Geometry check sheet. Reference: the model listing, model coordinates, mm. Face numbers are marked on the shaded views. A direction names the side the tool comes from. Give positions to 0.01 mm unless a question says otherwise; leave off trailing zeros. Loops run counter-clockwise (first coordinate to the right, second up) from the corner with the lowest first, then second, coordinate; pieces in that order, holes last. Notation, with made-up numbers: (2, 66) -> (21, 66) arc R17 cw to (21, 99) -> close; hole circle Ø4 at (89.5, -14.75). An arc over 180 degrees is marked (long way). Answer as a JSON object with one key per item and string values.
from build123d import *

# Parameters (mm, degrees)
SKETCH2_W           = 9.2
SKETCH2_H           = 22.44
SKETCH2_R           = 1.6
BOSS_EXTRUDE2_DEPTH = 3
SKETCH4_W           = 2
SKETCH4_H           = 22.44
BOSS_EXTRUDE3_DEPTH = 18
FILLET1_R           = 2
SKETCH5_R           = 1.6
CUT_EXTRUDE1_DEPTH  = 18


with BuildPart() as part:
    # Sketch2 → Boss-Extrude2 (new body)
    with BuildSketch(Plane(origin=(0, 0, 0), x_dir=(1, 0, 0), z_dir=(0, 1, 0))):
        with Locations((4.6, 11.22)):
            Rectangle(SKETCH2_W, SKETCH2_H)
        with Locations((5.6, 16.22)):
            Circle(SKETCH2_R, mode=Mode.SUBTRACT)
        with Locations((5.6, 6.22)):
            Circle(SKETCH2_R, mode=Mode.SUBTRACT)
    extrude(amount=BOSS_EXTRUDE2_DEPTH)

    # Sketch4 → Boss-Extrude3 (add)
    with BuildSketch(Plane(origin=(0, 3, 0), x_dir=(1, 0, 0), z_dir=(0, 1, 0))):
        with Locations((1, 11.22)):
            Rectangle(SKETCH4_W, SKETCH4_H)
    extrude(amount=BOSS_EXTRUDE3_DEPTH)

    # Fillet1
    fillet1_edges = [part.edges().sort_by_distance(p)[0] for p in [
        (0, 0, -11.22),
    ]]
    fillet(fillet1_edges, radius=FILLET1_R)

    # Sketch5 → Cut-Extrude1 (cut)
    with BuildSketch(Plane(origin=(2, 0, 0), x_dir=(0, 0, -1), z_dir=(1, 0, 0))):
        with Locations((2.42, 16)):
            Circle(SKETCH5_R)
        with Locations((20.02, 16)):
            Circle(SKETCH5_R)
    extrude(amount=-CUT_EXTRUDE1_DEPTH, mode=Mode.SUBTRACT)


solid = part.part
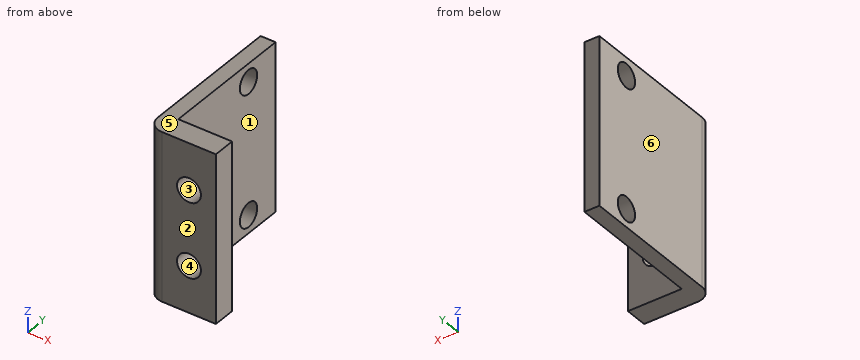
1) Section check D-D on z = -16.22. Record the cut outline in (x, y), plus the area to 3 significant figures.
Geometry check:
{"outline": "(0, 2) arc R2 ccw to (2, 0) -> (4, 0) -> (4, 3) -> (2, 3) -> (2, 21) -> (0, 21) -> close; (7.2, 0) -> (9.2, 0) -> (9.2, 3) -> (7.2, 3) -> close", "area": "53.1 mm2"}
2) Depth check by flat-ended pin: P1, Ø3, axis at x = 6, z = -9, coming from the +Y side; P2, Ø3, axis at y = 10.5, z = -13.5, coming from the +X side. Enter the tip coordinate at first touch or a pass-through.
Geometry check:
{"P1": "stops at y = 3", "P2": "stops at x = 2"}
3) Section check C-C on y = 16. Record the cut outline in (x, z), plus the area to 3 significant figures.
Geometry check:
{"outline": "(0, -22.44) -> (2, -22.44) -> (2, -21.62) -> (0, -21.62) -> close; (0, -18.42) -> (2, -18.42) -> (2, -4.02) -> (0, -4.02) -> close; (0, -0.82) -> (2, -0.82) -> (2, 0) -> (0, 0) -> close", "area": "32.1 mm2"}
4) Section check B-B on x = 5.6. Record the cut outline in (y, z), plus the area to 3 significant figures.
Geometry check:
{"outline": "(0, -22.44) -> (3, -22.44) -> (3, -17.82) -> (0, -17.82) -> close; (0, -14.62) -> (3, -14.62) -> (3, -7.82) -> (0, -7.82) -> close; (0, -4.62) -> (3, -4.62) -> (3, 0) -> (0, 0) -> close", "area": "48.1 mm2"}
5) Draft check along X on the marked faces 3, 4, 5 and 6. Enter one of: pulls with the +X half, pulls with the -X half, needs draft (parallel to the pull), parting line crosses it, or undercut.
Geometry check:
{"face 3": "undercut", "face 4": "undercut", "face 5": "needs draft", "face 6": "pulls with the -X half"}
6) Material ranges on line 1 along Z through (x, y) = (5.6, 1.8); line 2 along X through (y, z) = (2.35, -16.22); line 3 along X through (y, z) = (14, -11.25), recorded low to high. Write a range as from..to.
Geometry check:
{"line 1": "z = -22.44..-17.82, -14.62..-7.82, -4.62..0", "line 2": "x = 0..4, 7.2..9.2", "line 3": "x = 0..2"}
7) Tool access check on the marked faces 1 and 2. Record the directions out of +Z, -Z, +X, -X, +Y, -Y that give a thin tool (end or side, any length) a straight path to the whole face; none if there is none.
Geometry check:
{"face 1": "+Z, -Z, +X, +Y", "face 2": "+Z, -Z, +X, -X, -Y"}
8) Section check A-A on z = -20.02. Record the cut outline in (x, y), plus the area to 3 significant figures.
Geometry check:
{"outline": "(0, 2) arc R2 ccw to (2, 0) -> (9.2, 0) -> (9.2, 3) -> (2, 3) -> (2, 14.4) -> (0, 14.4) -> close; (0, 17.6) -> (2, 17.6) -> (2, 21) -> (0, 21) -> close", "area": "56.3 mm2"}
